Can you work these out from the drawing? Everything is in mm from the part's minimum corner. A direction names the side the tool comes from. Give positions to 0.01 mm unless a question says otherwise; leave off trailing zeros. Loops run counter-clockwise (first coordinate to the right, second up) from the corner with the lowest first, then second, coordinate; pieces in that order, holes last. Notation, with made-up numbers: (48.5, 80.25) - (107.5, 80.25) arc R20 ccw to (107.5, 107.25) - close; hole circle Ø1 at (-11.5, 75). An arc over 180 degrees is marked (long way). One line per item, written item: value. Start each with the question number.
Q1. If I drill on line 1 (X direction, y = 5.15, z = 4.5); line 2 (Z direction, x = 12.75, y = 5.15) (1 decimal); line 3 (Z direction, x = 12, y = 1.6) (1 decimal), over which ranges is the centre line in solid material (lowest first)? Write a range as from..to.
Q2. I want a section at C-C (z = 12.5). Please give me the cut outline in (x, y).
Q3. If we mould it in two halves opening along X, with no side actions, what happens to the marked faces 3, 4 and 5? For each: released by +X, released by -X, zero draft, split by the parting line, or undercut.
Q4. I'm going to push a flat-ended pin straight in: P1, Ø2, axis at x = 11.5, z = 13.5, coming from the +Y side. Where does the tip first touch, or does it pass through?
Q5. For the marked faces 1 and 2, which set-ups out of +Z, -Z, +X, -X, +Y, -Y let a thin tool reach every point of the face, with its end or its side?
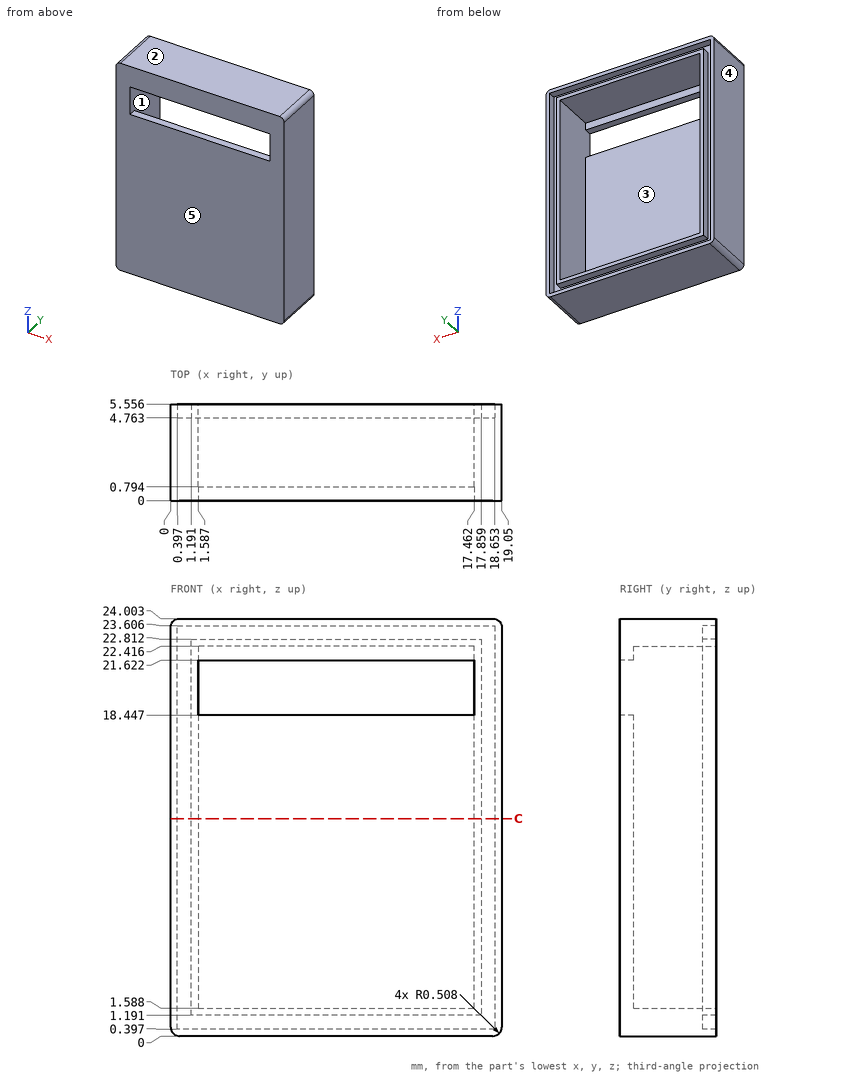
Worked answers:
1. line 1: x = 0..0.4, 1.19..1.59, 17.46..17.86, 18.65..19.05
1. line 2: z = 0..0.4, 1.2..1.6, 22.4..22.8, 23.6..24
1. line 3: z = 0..1.6, 22.4..24
2. outline: (0, 0) - (19.05, 0) - (19.05, 5.56) - (18.65, 5.56) - (18.65, 4.76) - (17.86, 4.76) - (17.86, 5.56) - (17.46, 5.56) - (17.46, 0.79) - (1.59, 0.79) - (1.59, 5.56) - (1.19, 5.56) - (1.19, 4.76) - (0.4, 4.76) - (0.4, 5.56) - (0, 5.56) - close
3. face 3: undercut
3. face 4: released by -X
3. face 5: zero draft
4. P1: stops at y = 0.79
5. face 1: +Y
5. face 2: +Z, +X, -X, +Y, -Y
